Can you work these out from the model? Positions are in its coordinate system, mm. Give positions to 0.01 mm unless a question says otherwise; leave off trailing zeros. Loops run counter-clockwise (first coordinate to the right, second up) from the corner with the lowest first, then second, coordinate; pieces in that order, holes last. Notation, with made-up numbers: M 4.25,88 L 10.25,88 A13 cw 10.25,105 Z; hole C 73.5,38.5 d9. An arc over 180 degrees is marked long. Answer as a JSON object with one key per item and string values.
Autodesk Inventor part; units mm, degrees
ref_plane "YZ Plane" through (0, 0, 0) normal (1, 0, 0) x (0, 1, 0)
ref_plane "XZ Plane" through (0, 0, 0) normal (0, 1, 0) x (-1, 0, 0)
ref_plane "XY Plane" through (0, 0, 0) normal (0, 0, 1) x (1, 0, 0)
sketch "スケッチ1" plane through (0, 0, 0) normal (0, 0, 1) x (1, 0, 0)
  line L0 (-5, 12) -> (5, 12)
  line L1 (5, 12) -> (5, 0)
  line L2 (5, 0) -> (-5, 0)
  line L3 (-5, 0) -> (-5, 12)
  line L4 (-8.0749, 12) -> (-5, 12) construction
  point P0 (0, 0)
  point P1 (0, 12)
  point P2 (0, 0)
  dimension "d0" = 12
  dimension "d1" = 10
  dimension "d2" = 10
extrude "押し出し1" add sketch "スケッチ1" along normal blind 3
sketch "スケッチ2" plane through (-5, 12, 0) normal (0, 1, 0) x (1, 0, 0)
  line L0 (0, -3) -> (10, -3)
  line L1 (0, 0) -> (10, 0)
  line L2 (2.5173, -3) -> (0, 0)
  line L3 (10, 0) -> (7.4827, -3)
  line L4 (0, 0) -> (0, -3)
  line L5 (10, 0) -> (10, -3)
  point P0 (5, 0)
  dimension "d5" = 80
  dimension "d6" = 40
  dimension "d7" = 40
extrude "押し出し2" cut sketch "スケッチ2" against normal through all contours L4 L2 L0 | L3 L5 L0
sketch "スケッチ3" plane through (-5, 0, 0) normal (-0.766, 0, 0.6428) x (0.6428, 0, 0.766)
  line L0 (3.9162, 0) -> (0, 0)
  line L1 (3.9162, 12) -> (3.9162, 0)
  line L2 (0, 12) -> (3.9162, 12)
  line L3 (0, 12) -> (0, 0)
  line L4 (3.9162, 0) -> (7.1079, 0)
  line L5 (3.9162, 0) -> (-11.0838, 7)
  point P0 (3.2139, 0)
  point P1 (0, 1.8276)
  dimension "d10" = 15
  dimension "d11" = 7
extrude "押し出し3" cut sketch "スケッチ3" against normal through all contours L0 L3 L5
sketch "スケッチ4" plane through (5, 0, 0) normal (0.766, 0, 0.6428) x (0.6428, 0, -0.766)
  line L0 (0, 0) -> (-3.9162, 0)
  line L1 (0, 0) -> (0, 12)
  line L2 (-3.9162, 12) -> (0, 12)
  line L3 (-3.9162, 0) -> (-3.9162, 12)
  line L4 (-3.9162, 0) -> (11.0838, 7)
  point P0 (-3.2139, 0)
  point P1 (0, 1.8276)
  dimension "d14" = 15
  dimension "d15" = 7
extrude "押し出し4" cut sketch "スケッチ4" against normal through all contours L0 L4 L1
sketch "スケッチ13" plane through (-5, 1.8276, 0) normal (-0.766, 0, 0.6428) x (0.6428, 0, 0.766)
  circle A0 centre (2.4162, 8.1724) radius 0.8
  circle A1 centre (2.4162, 1.1724) radius 0.8
  point P0 (3.2139, -1.8276)
extrude "押し出し13" cut sketch "スケッチ13" against normal through all
mirror "ミラー1" about plane through (0, 0, 0) normal (1, 0, 0) of "押し出し13"
sketch "スケッチ15" plane through (0, 0, 3) normal (0, 0, 1) x (1, 0, 0)
  line L0 (-2.4827, 0) -> (2.4827, 0)
  line L1 (2.4827, 12) -> (-2.4827, 12)
  circle A0 centre (0, 4) radius 0.8
  circle A1 centre (0, 8) radius 0.8
  point P0 (0, 0)
  point P1 (0, 0)
  dimension "d44" = 1.6
  dimension "d45" = 1.6
  dimension "d46" = 4
  dimension "d47" = 4
  dimension "d49" = 4
extrude "押し出し14" cut sketch "スケッチ15" against normal through all
equation "\"d6\" = d7"
equation "\"d47\" = d49"
properties part number "antana_middle"
1) Suppose I cut it at A-A, the plane y = 4.5. Write out the boundary of the cut face in (x, z), and give its area (3 significant figures).
Answer list:
{"outline": "M -5,0 L -0.62,0 L -0.62,3 L -2.48,3 Z; M 0.62,0 L 5,0 L 2.48,3 L 0.62,3 Z", "area": "18.7 mm^2"}
2) Suppose I cut it at C-C, the plane y = 8. Write out the boundary of the cut face in (x, z), and give its area (3 significant figures).
Answer list:
{"outline": "M -5,0 L -0.8,0 L -0.8,3 L -2.48,3 Z; M 0.8,0 L 5,0 L 2.48,3 L 0.8,3 Z", "area": "17.6 mm^2"}
3) Will these pins go through, and if not, where does the flat tip stop? pin 1 Ø5 at (x, y) = (3, 10) entering from +Z; pin 2 Ø1.5 at (y, z) = (7, 1) entering from +X.
Answer list:
{"pin 1": "z = 3", "pin 2": "x = 4.79"}
4) If we mould it in two halves opening along Z, with no side actions, what happens to faces 1 (the cylindrical face through (-0.104, 4.793, 1.521)), 2 (the cylindrical face through (-1.84, 3.24, 1.5)), 3 (the flat face through (3.76, 6.08, 1.48))? For each: +Z half, -Z half, draft (parallel to the pull), parting line (faces both ways), or undercut.
Answer list:
{"face 1": "draft", "face 2": "undercut", "face 3": "+Z half"}
5) Please list where these lines run through material, in increasing order: line 1 along Y through (x, z) = (0, 1.6); line 2 along Y through (x, z) = (0, 0.75); line 3 along X through (y, z) = (3.5, 1.15). Write a range as from..to.
Answer list:
{"line 1": "0..3.2, 4.8..7.2, 8.8..12", "line 2": "0.06..3.2, 4.8..7.2, 8.8..12", "line 3": "-4.04..-3.58, -1.64..-0.62, 0.62..1.64, 3.58..4.04"}
6) Suppose I cut it at B-B, the plane y = 9.5. Write out the boundary of the cut face in (x, z), and give its area (3 significant figures).
Answer list:
{"outline": "M -5,0 L -2.21,0 L -3.85,1.37 Z; M -3.05,2.33 L -0.27,0 L 0.27,0 L 3.05,2.33 L 2.48,3 L -2.48,3 Z; M 2.21,0 L 5,0 L 3.85,1.37 Z", "area": "15.3 mm^2"}
7) Suppose I cut it at D-D, the plane z = 0.7. Give the number of separate pieces and of enclosed holes in the cut face, and give its area (3 significant figures).
Answer list:
{"separate pieces": "1", "enclosed holes": "6", "area": "82.8 mm^2"}
